Check sheet for the modelled part. Datum: model origin and axes. Units: mm. Round coordinates to 2 decimals unless told otherwise and drop trailing zeros. Loops run counter-clockwise (first coordinate to the right, second up) from the corner with the lowest first, then second, coordinate; pieces in that order, holes last. Notation, with made-up numbers: (26.5, -21.75) - (47.5, -21.75) arc R24 cw to (47.5, 11.25) - close; hole circle Ø10 at (37, -37). An arc over 180 degrees is marked (long way). Put each result on its own line as item: value. Start each with the question number.
Item 1: Section check A-A, the plane y = 299. Record the cut outline in (x, z), and give its area (3 significant figures).
Item 2: Section check D-D, the plane z = 0. Record the cut outline in (x, y).
Item 3: Section check C-C, the plane y = 220. Record the cut outline in (x, z), and give its area (3 significant figures).
Item 4: Section check B-B, the plane x = 200. Record the cut outline in (y, z), and give its area (3 significant figures).
Item 5: Material ranges on line 1 along Y through (x, z) = (109, -139); line 2 along Z through (x, y) = (-63, 154.5); line 3 along X through (y, z) = (33.5, 123), recorded low to high.
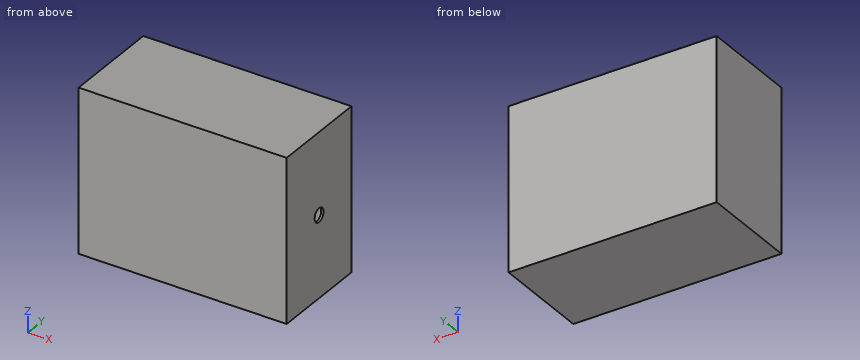
from build123d import *

# Parameters (mm, degrees)
SKETCH1_W           = 920
SKETCH1_H           = 720
BOSS_EXTRUDE1_DEPTH = 440
SHELL1_T            = 10
CUT_EXTRUDE1_REACH  = 922
SKETCH2_R           = 30.075332342


with BuildPart() as part:
    # Sketch1 → Boss-Extrude1 (new body)
    with BuildSketch(Plane(origin=(0, 0, 0), x_dir=(1, 0, 0), z_dir=(0, 1, 0))):
        Rectangle(SKETCH1_W, SKETCH1_H)
    extrude(amount=BOSS_EXTRUDE1_DEPTH)

    # Shell1 (no face opened: a closed hollow body)
    add(offset(amount=-SHELL1_T, mode=Mode.PRIVATE), mode=Mode.SUBTRACT)

    # Sketch2 → Cut-Extrude1 (cut, up to next)
    with BuildSketch(Plane(origin=(460, 0, 0), x_dir=(0, 0, -1), z_dir=(1, 0, 0)), mode=Mode.PRIVATE) as cut_extrude1_sk1:
        with Locations((0, 220)):
            Circle(SKETCH2_R)
    cut_extrude1_tool1 = extrude(cut_extrude1_sk1.sketch, amount=-CUT_EXTRUDE1_REACH, mode=Mode.PRIVATE) & part.part
    add(cut_extrude1_tool1.solids().sort_by_distance((460, 220, 0))[0], mode=Mode.SUBTRACT)


solid = part.part
Check result:
1. outline: (-460, -360) - (460, -360) - (460, 360) - (-460, 360) - close; hole (-450, -350) - (450, -350) - (450, 350) - (-450, 350) - close
1. area: 32,400 mm²
2. outline: (-460, 0) - (460, 0) - (460, 189.92) - (450, 189.92) - (450, 10) - (-450, 10) - (-450, 430) - (450, 430) - (450, 250.08) - (460, 250.08) - (460, 440) - (-460, 440) - close
3. outline: (-460, -360) - (460, -360) - (460, -30.08) - (450, -30.08) - (450, -350) - (-450, -350) - (-450, 350) - (450, 350) - (450, 30.08) - (460, 30.08) - (460, 360) - (-460, 360) - close
3. area: 31,800 mm²
4. outline: (0, -360) - (440, -360) - (440, 360) - (0, 360) - close; hole (10, -350) - (430, -350) - (430, 350) - (10, 350) - close
4. area: 22,800 mm²
5. line 1: 0 to 10, 430 to 440
5. line 2: -360 to -350, 350 to 360
5. line 3: -460 to -450, 450 to 460
